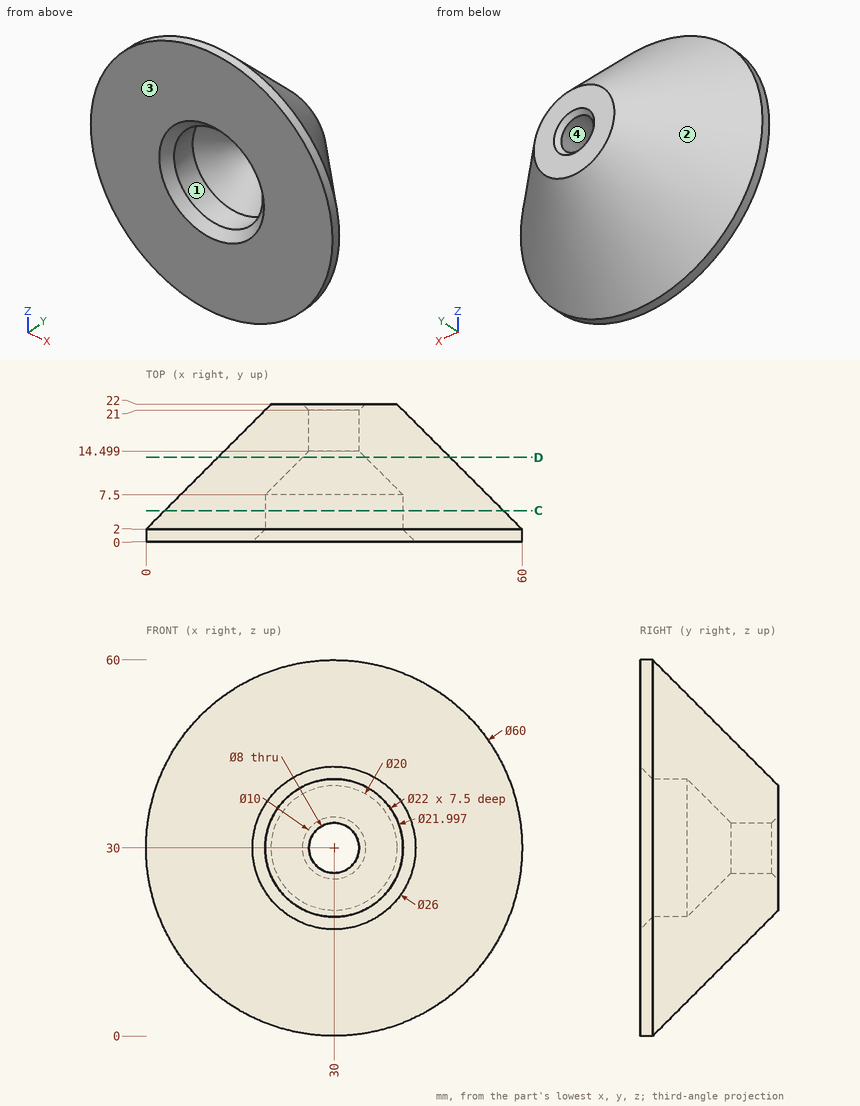
Input: dimensioned drawing with shaded views. Units: mm. Origin: part minimum x, y, z. Give positions to 0.01 mm unless a question says otherwise; leave off trailing zeros. Write each loop counter-clockwise with the first axis right and the second up, starting at its lowest first coordinate (ties: lowest second). Pieces come first, ordered by that corner, then holes.
1. Section query C-C (y = 5). Return the cut outline in (x, z).
2. Material intervals for line 1 along Z through (x, y) = (30, 3.3); line 2 along X through (y, z) = (17.5, 30); line 3 along X through (y, z) = (3.8, 30), sorted ascending.
3. First-contact query: pin 1 (2 mm diameter, centred on x = 27, y = 10, fed in from +Z); pin 2 (1.5 mm diameter, centred on x = 46, y = 9.5, fed in from +Z) (1 decimal); pin 3 (8 mm diameter, centred on x = 51, y = 8, fed in from -Z); pin 4 (8 mm diameter, centred on x = 53, z = 51, fed in from -Y). Flat tips, straight axial feed; report the tip coordinate or a pass-through.
4. Pull-direction query (Z, two-part tool) for the marked faces 1, 2, 3 and 4; classes: +Z half, -Z half, draft (parallel to the pull), parting line (faces both ways), or undercut.
5. Section query D-D (y = 13.5). Return the cut outline in (x, z).
Output values:
1. outline: circle Ø54 at (30, 30); hole circle Ø22 at (30, 30)
2. line 1: z = 1.3 to 19, 41 to 58.7
2. line 2: x = 15.5 to 26, 34 to 44.5
2. line 3: x = 1.8 to 19, 41 to 58.2
3. pin 1: stops at z = 52.81
3. pin 2: stops at z = 47.1
3. pin 3: stops at z = 10.15
3. pin 4: stops at y = 0
4. face 1: undercut
4. face 2: parting line
4. face 3: draft
4. face 4: undercut
5. outline: circle Ø37 at (30, 30); hole circle Ø10 at (30, 30)
